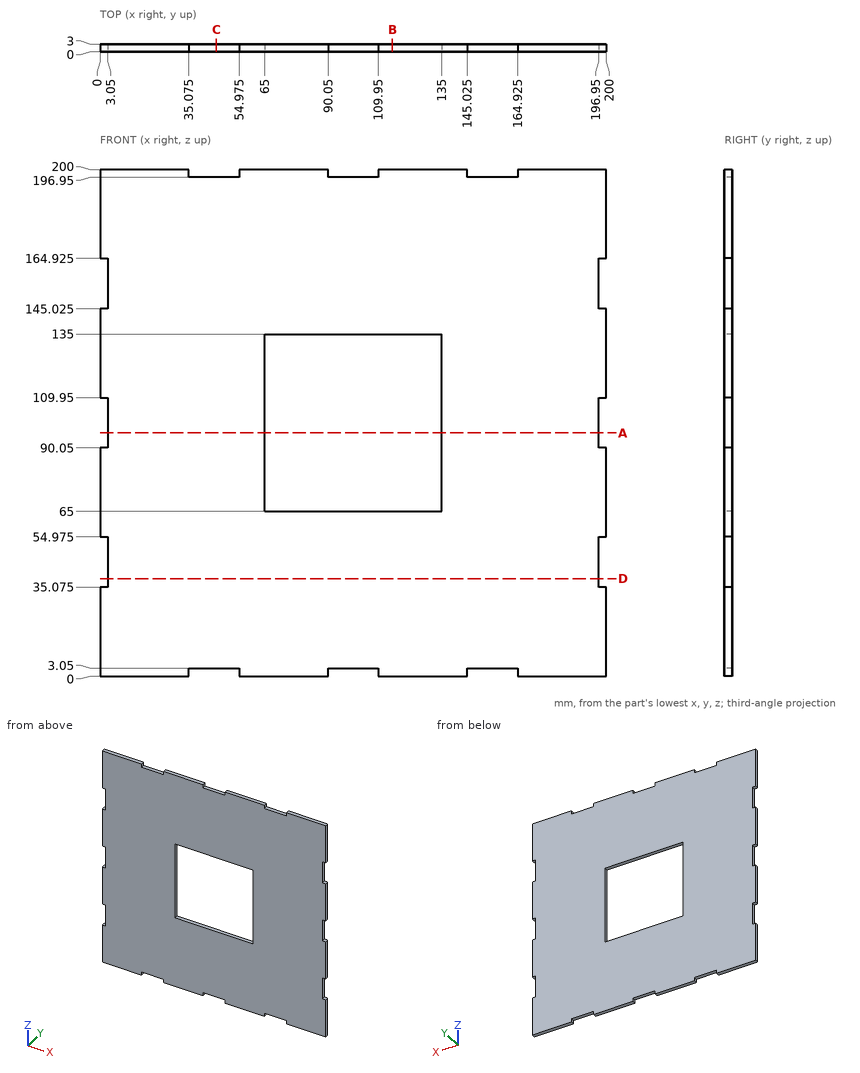
Print and shaded views of the part. All mm, measured from the part's lowest x, y and z. Round coordinates to 2 decimals unless told otherwise and drop trailing zeros. Write each loop counter-clockwise with the first axis right and the second up, starting at its lowest first coordinate (ties: lowest second). Pieces come first, ordered by that corner, then holes. Notation, with made-up numbers: (36.25, -18) -> (85.25, -18) arc R10 cw to (85.25, -1) -> close; hole circle Ø5 at (0.5, 76). An arc over 180 degrees is marked (long way). Return JSON: item names as keys, results as strings. Group by question number.
Q1. Pin check, flat tips, straight feed: pin 1 (0.9 mm diameter, centred on y = 1.5, z = 198.5, fed in from -X); pin 2 (1.5 mm diameter, centred on x = 49, y = 2, fed in from +Z); pin 3 (1.5 mm diameter, centred on x = 101.5, y = 1.5, fed in from -Z); pin 4 (0.9 mm diameter, centred on y = 2, z = 160, fed in from +X). Stop position of each tip, or through.
Q2. Saw through at D-D on z = 38.5. Write the cut outline in (x, y).
Q3. Saw through at B-B on x = 115.5. Write the cut outline in (y, z), plus the area to 3 significant figures.
Q4. Probe L1, parallel to X at y = 2.7, z = 78.5; L2, parallel to Z at x = 109, y = 1.55. List the from-to ranges inside material, lowest first. Write a range as [from, to].
Q5. Saw through at A-A on z = 96. Write the cut outline in (x, y), plus the area to 3 significant figures.
Q6. Saw through at C-C on x = 46. Write the cut outline in (y, z), plus the area to 3 significant figures.
Answer:
{
 "1": {"pin 1": "x = 0", "pin 2": "z = 196.95", "pin 3": "z = 3.05", "pin 4": "x = 196.95"},
 "2": {"outline": "(3.05, 0) -> (196.95, 0) -> (196.95, 3) -> (3.05, 3) -> close"},
 "3": {"outline": "(0, 0) -> (3, 0) -> (3, 65) -> (0, 65) -> close; (0, 135) -> (3, 135) -> (3, 200) -> (0, 200) -> close", "area": "390 mm2"},
 "4": {"L1": "[0, 65], [135, 200]", "L2": "[3.05, 65], [135, 196.95]"},
 "5": {"outline": "(3.05, 0) -> (65, 0) -> (65, 3) -> (3.05, 3) -> close; (135, 0) -> (196.95, 0) -> (196.95, 3) -> (135, 3) -> close", "area": "372 mm2"},
 "6": {"outline": "(0, 3.05) -> (3, 3.05) -> (3, 196.95) -> (0, 196.95) -> close", "area": "582 mm2"}
}
